Autodesk Inventor part; units mm, degrees
ref_plane "YZ Plane" through (0, 0, 0) normal (1, 0, 0) x (0, 1, 0)
ref_plane "XZ Plane" through (0, 0, 0) normal (0, 1, 0) x (-1, 0, 0)
ref_plane "XY Plane" through (0, 0, 0) normal (0, 0, 1) x (1, 0, 0)
sketch "Sketch1" plane through (0, 0, 0) normal (0, 0, 1) x (1, 0, 0)
  line L0 (-12.7, -12.7) -> (12.7, -12.7)
  line L1 (12.7, -12.7) -> (12.7, 12.7)
  line L2 (12.7, 12.7) -> (-12.7, 12.7)
  line L3 (-12.7, 12.7) -> (-12.7, -12.7)
  line L4 (-11.1125, -11.1125) -> (11.1125, -11.1125)
  line L5 (11.1125, -11.1125) -> (11.1125, 11.1125)
  line L6 (11.1125, 11.1125) -> (-11.1125, 11.1125)
  line L7 (-11.1125, 11.1125) -> (-11.1125, -11.1125)
  point P0 (0, 0)
  dimension "d0" = 25.4
  dimension "d1" = 25.4
  dimension "d2" = 22.225
  dimension "d3" = 22.225
extrude "Extrusion1" add sketch "Sketch1" along normal blind 203.2
equation "\"BendRadius\" = Thickness"
equation "\"BendReliefWidth\" = Thickness"
equation "\"BendReliefDepth\" = 0.5 * Thickness"
equation "\"CornerReliefSize\" = 4 * Thickness"
equation "\"MinimumRemnant\" = 2 * Thickness"
equation "\"TransitionRadius\" = BendRadius"
equation "\"JacobiRadiusSize\" = BendRadius"
equation "\"GapSize\" = Thickness"
properties part number "8 in 1-16"
Geometry: final body of the model. Coordinates: model frame, mm. A direction names the side the tool comes from. Give positions to 0.01 mm unless a question says otherwise; leave off trailing zeros. Write each loop counter-clockwise with the first axis right and the second up, starting at its lowest first coordinate (ties: lowest second). Pieces come first, ordered by that corner, then holes.
(1) Access query for faces 4 (the flat face through (12.7, 0, 100)), 5 (the flat face through (-11.112, 0, 100)). Directions: +Z, -Z, +X, -X, +Y, -Y. A direction counts if a zero-diameter tool reaches every point of the face in a straight line with its end or side. Return the directions, or none.
(2) Cut plane C-C, the plane z = 156. Return loops of the section in (x, y), then the cut area to 3 significant figures.
(3) Mould query, pull axis Y, two halves, no side actions, for faces 1 (the flat face through (-11.3, 0.1, 203.2)), 2 (the flat face through (0, 12.7, 100)), 3 (the flat face through (0, -11.112, 100)). Classes: released by +Y, released by -Y, zero draft, split by the parting line, or undercut.
(4) Ray query, line 1 (Y direction, x = 8.75, z = 188.5). Return the intervals inside material, ascending.
(5) Cut plane A-A, the plane x = 4.5. Return loops of the section in (y, z), then the cut area to 3 significant figures.
Values follow:
1. face 4: +Z, -Z, +X, +Y, -Y
1. face 5: +Z, -Z
2. outline: (-12.7, -12.7) - (12.7, -12.7) - (12.7, 12.7) - (-12.7, 12.7) - close; hole (-11.11, -11.11) - (11.11, -11.11) - (11.11, 11.11) - (-11.11, 11.11) - close
2. area: 151 mm2
3. face 1: zero draft
3. face 2: released by +Y
3. face 3: undercut
4. line 1: y = -12.7 to -11.11, 11.11 to 12.7
5. outline: (-12.7, 0) - (-11.11, 0) - (-11.11, 203.2) - (-12.7, 203.2) - close; (11.11, 0) - (12.7, 0) - (12.7, 203.2) - (11.11, 203.2) - close
5. area: 645 mm2
